Here's how the part is built. I have some questions about the finished solid (model axes, mm). A direction names the side the tool comes from. Round coordinates to 2 decimals unless told otherwise and drop trailing zeros. Write each loop counter-clockwise with the first axis right and the second up, starting at its lowest first coordinate (ties: lowest second). Pieces come first, ordered by that corner, then holes. Notation, with made-up numbers: (19.5, 59) -> (43.5, 59) arc R16 ccw to (43.5, 78) -> close; hole circle Ø3 at (80, -38.5). An arc over 180 degrees is marked (long way). Answer as CSV lines item,"result".
```python
from build123d import *

# Parameters (mm, degrees)
CHAMFER1_SIZE           = 0.508
SKETCH2_W               = 19.211267794
SKETCH2_H               = 1.27
BOSS_EXTRUDE1_DEPTH     = 80.01
FILLET1_R               = 0.127
CUT_EXTRUDE1_DEPTH      = 82.521536431
CUT_EXTRUDE1_DEPTH_BACK = 82.521536431
SKETCH3_R               = 0.5334


with BuildPart() as part:
    # Sketch1 → Revolve1 (revolve)
    with BuildSketch(Plane.XY, mode=Mode.PRIVATE) as revolve1_sk:
        Polygon((0, 13.97), (-11.049, 13.97), (-11.049, 11.43), (-10.1346, 11.43), (-10.1346, 9.398), (-8.89, 9.398), (-8.89, 6.985), (-10.1346, 6.985), (-10.1346, 5.207), (-8.89, 5.207), (-8.89, 2.794), (-10.1346, 2.794), (-10.1346, 0), (0, 0), align=None)
    revolve(revolve1_sk.sketch.rotate(Axis((0, 20.368840099, 0), (0, -1, 0)), 270), axis=Axis((0, 20.368840099, 0), (0, -1, 0)))

    # Chamfer1
    chamfer1_edges = [part.edges().sort_by_distance(p)[0] for p in [
        (0, 0, -10.1346),
    ]]
    chamfer(chamfer1_edges, length=CHAMFER1_SIZE)

    # Sketch2 → Boss-Extrude1 (add)
    with BuildSketch(Plane.XZ):
        Rectangle(SKETCH2_W, SKETCH2_H)
    extrude(amount=BOSS_EXTRUDE1_DEPTH)

    # Fillet1
    fillet1_edges = [part.edges().sort_by_distance(p)[0] for p in [
        (0, 11.43, -10.1346),
    ]]
    fillet(fillet1_edges, radius=FILLET1_R)

    # Sketch3 → Cut-Extrude1 (cut, two sides: drawn at the far end of the back side and taken through both)
    with BuildSketch(Plane(origin=(0, 0, 0), x_dir=(0, 0, -1), z_dir=(1, 0, 0)).offset(-CUT_EXTRUDE1_DEPTH_BACK)):
        with Locations((0, 10.414)):
            Circle(SKETCH3_R)
    extrude(amount=CUT_EXTRUDE1_DEPTH + CUT_EXTRUDE1_DEPTH_BACK, mode=Mode.SUBTRACT)


solid = part.part
```
1. Suppose I cut it at B-B on y = -22. Please give me the cut outline in (x, z) (3 decimals), and give its area (3 significant figures).
Numbers:
outline,"(-9.606, -0.635) -> (9.606, -0.635) -> (9.606, 0.635) -> (-9.606, 0.635) -> close"
area,"24.4 mm^2"
2. On a 3-axis mill with a long thin cutter (end or side, diameter ignored), from which of +Z, -Z, +X, -X, +Y, -Y can I reach the whole of each face in a straight line? I mean faces 1 (the face through (-3.04, 10.34, 9.67)), 2 (the face through (0, -39, -0.635)), 3 (the face through (9, 9.398, 1)). Say none if no direction works.
Numbers:
face 1,"-Y"
face 2,"-Z, +X, -X, -Y"
face 3,"none"
3. If we mould it in two halves opening along Y, with no side actions, what happens to faces 4 (the face through (8.68, 3.98, -1.93)), 5 (the face through (0, 13.97, 0)), 6 (the face through (-3.04, 1.63, 9.67))? For each: released by +Y, released by -Y, zero draft, split by the parting line, or undercut.
Numbers:
face 4,"undercut"
face 5,"released by +Y"
face 6,"zero draft"
4. For pin 1 Ø4.5 at (x, z) = (1, 4.5) entering from -Y; pin 2 Ø6 at (x, y) = (-3.5, -39) entering from -Z (3 decimals); pin 3 Ø1.5 at (x, y) = (-8.5, -49) entering from +Z (3 decimals), each with a flat end and sliding along its axis, tell me the tip position at first contact or that it passes through.
Numbers:
pin 1,"stops at y = 0"
pin 2,"stops at z = -0.635"
pin 3,"stops at z = 0.635"
5. If I drill on line 1 (Y direction, x = -2.5, z = 9.5) (3 decimals); line 2 (Y direction, x = 0.75, z = 0); line 3 (Y direction, x = -3.25, z = -9.5) (3 decimals), over which ranges is the centre line in solid material (lowest first)?
Numbers:
line 1,"y = 0.197 to 2.794, 5.207 to 6.985, 9.398 to 13.97"
line 2,"y = -80.01 to 9.88, 10.95 to 13.97"
line 3,"y = 0.414 to 2.794, 5.207 to 6.985, 9.398 to 13.97"
